Here's how the part is built. I have some questions about the finished solid (model axes, mm). A direction names the side the tool comes from. Give positions to 0.01 mm unless a question says otherwise; leave off trailing zeros. Loops run counter-clockwise (first coordinate to the right, second up) from the corner with the lowest first, then second, coordinate; pieces in that order, holes last. Notation, with made-up numbers: (30.25, 55.5) -> (45.25, 55.5) arc R16 ccw to (45.25, 72.5) -> close; hole circle Ø3 at (-19, 9). An arc over 180 degrees is marked (long way). Answer in a Markdown table with one row per item. Add a question column.
Item 1: Which directions (+Z, -Z, +X, -X, +Y, -Y) give clear straight access to the entire face, cutting with the end or side of a thin tool? Please do faces 1 (the face through (1, 12, -22)), 2 (the face through (1, 12, -2)), 3 (the face through (1, 0, -12)).
Item 2: If we section it at D-D (z = -20.5): Write out the boundary of the cut face in (x, y).
Item 3: If we section it at B-B (y = 10.25): Write out the boundary of the cut face in (x, z), then the cut area to 3 significant figures.
Item 4: For P1, Ø1.5, axis at x = 4.5, z = -16.5, coming from the +Y side; P2, Ø1, axis at x = 1, z = -2.5, coming from the -Y side; P3, Ø1.5, axis at x = 3, z = -6.5, coming from the +Y side; P4, Ø0.8, axis at y = 0, z = -19, coming from the -X side, each with a flat end and sliding along its axis, tell me the tip position at first contact or that it passes through.
Item 5: If we section it at C-C (x = 7.5): Write out the boundary of the cut face in (y, z).
Item 6: We'd pull the mould along Y, two halves only. Please class faces 4 (the face through (5.944, 8.314, -17.542)), 5 (the face through (1, 9, 0)), 6 (the face through (1, 5.5, 0)): released by +Y, released by -Y, zero draft, split by the parting line, or undercut.
Item 7: If I drill on line 1 (Z direction, x = 1.5, y = 6); line 2 (X direction, y = 3.75, z = -18.25); line 3 (Y direction, x = 1.75, z = -22.5), over which ranges is the centre line in solid material (lowest first)?
Autodesk Inventor part; units mm, degrees
ref_plane "YZ Plane" through (0, 0, 0) normal (1, 0, 0) x (0, 1, 0)
ref_plane "XZ Plane" through (0, 0, 0) normal (0, 1, 0) x (-1, 0, 0)
ref_plane "XY Plane" through (0, 0, 0) normal (0, 0, 1) x (1, 0, 0)
sketch "Náčrt1" plane through (0, 0, 0) normal (1, 0, 0) x (0, 1, 0)
  arc A0 (12, -4) -> (12, -6) centre (12, -5) ccw
  arc A1 (0, -6.1587) -> (0, -4.1587) centre (0, -5.1587) ccw
  arc A2 (12, -20) -> (12, -18) centre (12, -19) ccw
  arc A3 (0, -18) -> (0, -20) centre (0, -19) ccw
  line L0 (0, -4.1587) -> (0, 0)
  line L1 (12, 0) -> (12, -4)
  line L2 (12, -6) -> (12, -18)
  line L3 (12, -20) -> (12, -24)
  line L4 (0, -24) -> (0, -20)
  line L5 (0, -18) -> (0, -6.1587)
  circle A4 centre (12, -19) radius 0.5002
  circle A5 centre (0, -19) radius 0.5002
  arc A6 (7, 0) -> (5, 0) centre (6, 0) ccw
  line L6 (0, 0) -> (5, 0)
  line L7 (7, 0) -> (12, 0)
  circle A7 centre (6, 0) radius 0.5
  arc A8 (7, -24) -> (5, -24) centre (6, -24) ccw
  line L8 (12, -24) -> (7, -24)
  line L9 (5, -24) -> (0, -24)
  dimension "d0" = 12
  dimension "d1" = 24
  dimension "d2" = 2
  dimension "d3" = 2
  dimension "d4" = 5
  dimension "d5" = 5
  dimension "d6" = 5
  dimension "d7" = 2
  dimension "d8" = 1
extrude "Vysunutí1" add sketch "Náčrt1" along normal blind 2
sketch "Náčrt2" plane through (2, 0, 0) normal (1, 0, 0) x (0, 0, -1)
  circle A0 centre (12, 6.016) radius 6
  arc A1 (24, 7) -> (24, 5) centre (24, 6) ccw
  point P0 (0, 0)
  dimension "d11" = 12
  dimension "d12" = 12
extrude "Vysunutí2" add sketch "Náčrt2" along normal blind 8
equation "\"d6\" = d5"
properties part number "Grove - Oxygen Sensor"
Recorded:
| question | item | result |
|---|---|---|
| 1 | face 1 | -Z, +X, -X, +Y |
| 1 | face 2 | +Z, +X, -X, +Y |
| 1 | face 3 | +Z, +X, -X, -Y |
| 2 | outline | (0, 0) -> (2, 0) -> (2, 12) -> (0, 12) -> close |
| 3 | outline | (0, -24) -> (2, -24) -> (2, -16.25) -> (10, -16.25) -> (10, -7.75) -> (2, -7.75) -> (2, 0) -> (0, 0) -> close |
| 3 | area | 116 mm^2 |
| 4 | P1 | stops at y = 10.7 |
| 4 | P2 | stops at y = 0 |
| 4 | P3 | stops at y = 9.68 |
| 4 | P4 | passes through |
| 5 | outline | circle Ø12 at (6.02, -12) |
| 6 | face 4 | split by the parting line |
| 6 | face 5 | zero draft |
| 6 | face 6 | undercut |
| 7 | line 1 | z = -23 to -0.5, 0.5 to 1 |
| 7 | line 2 | x = 0 to 2 |
| 7 | line 3 | y = 0 to 12 |
